from build123d import *

# Parameters (mm, degrees)
SKETCH_1_W      = 470
SKETCH_1_H      = 180
SKETCH_1_R      = 1.5
SKETCH_1_R_2    = 7
SKETCH_1_R_3    = 2
SKETCH_1_W_2    = 185
SKETCH_1_H_2    = 143
EXTRUDE_1_DEPTH = 5


with BuildPart() as part:
    # 草图1 → 凸台-拉伸1 (new body)
    with BuildSketch(Plane(origin=(0, 0, 0), x_dir=(1, 0, 0), z_dir=(0, 1, 0))):
        with Locations((0, 15)):
            Rectangle(SKETCH_1_W, SKETCH_1_H)
        with Locations((-96.5, 86)):
            Circle(SKETCH_1_R, mode=Mode.SUBTRACT)
        with Locations((96.5, 86)):
            Circle(SKETCH_1_R, mode=Mode.SUBTRACT)
        with Locations((96.5, -56)):
            Circle(SKETCH_1_R, mode=Mode.SUBTRACT)
        with Locations((-96.5, -56)):
            Circle(SKETCH_1_R, mode=Mode.SUBTRACT)
        with Locations((-125, 75)):
            Circle(SKETCH_1_R_2, mode=Mode.SUBTRACT)
        with Locations((-125, 45)):
            Circle(SKETCH_1_R_2, mode=Mode.SUBTRACT)
        with Locations((-125, 15)):
            Circle(SKETCH_1_R_2, mode=Mode.SUBTRACT)
        with Locations((-125, -15)):
            Circle(SKETCH_1_R_2, mode=Mode.SUBTRACT)
        with Locations((-125, -45)):
            Circle(SKETCH_1_R_2, mode=Mode.SUBTRACT)
        with Locations((-226, 35)):
            Circle(SKETCH_1_R, mode=Mode.SUBTRACT)
        with Locations((-186, 35)):
            Circle(SKETCH_1_R, mode=Mode.SUBTRACT)
        with Locations((-186, -5)):
            Circle(SKETCH_1_R, mode=Mode.SUBTRACT)
        with Locations((-226, -5)):
            Circle(SKETCH_1_R, mode=Mode.SUBTRACT)
        with Locations((-210, -50)):
            Circle(SKETCH_1_R_3, mode=Mode.SUBTRACT)
        with Locations((210, -50)):
            Circle(SKETCH_1_R_3, mode=Mode.SUBTRACT)
        with Locations((-210, 80)):
            Circle(SKETCH_1_R_3, mode=Mode.SUBTRACT)
        with Locations((210, 80)):
            Circle(SKETCH_1_R_3, mode=Mode.SUBTRACT)
        with Locations((0, 15)):
            Rectangle(SKETCH_1_W_2, SKETCH_1_H_2, mode=Mode.SUBTRACT)
    extrude(amount=EXTRUDE_1_DEPTH)


solid = part.part
Work out the finished part from the listing and answer in its coordinate system (mm). Round coordinates to 2 decimals unless told otherwise and drop trailing zeros. Order: outer loops, then holes, each group sorted by start corner. A loop starts at its lowest first (then second) coordinate and runs counter-clockwise, first axis right, second up. Notation, with made-up numbers: M -21,66 L -13,66 A10 ccw -13,82 Z; hole C -26.5,16 d7. An arc over 180 degrees is marked long. Put each result on its own line as item: value. Start each with the question number.
Q1. A flat-ended cylindrical pin translates along its axis: pin 1 (5 mm diameter, centred on x = 110.5, z = 35.5, fed in from -Y). Find the tip coordinate at first contact, or state that the pin passes through.
Q2. Section C-C, the plane y = 1.1 is taken. Give the number of separate pieces and of enclosed holes in the cut face, and give its area (3 significant figures).
Q3. Straight lines are drawn through the part: L1, parallel to X at y = 3.85, z = -86; L2, parallel to Z at x = 96.5, y = 1.25; L3, parallel to X at y = 2.65, z = 15. For each, find the intervals that lie inside material, in ascending order. Write a range as [from, to].
Q4. Section A-A, the plane z = 15 is taken. Write down the section's boundary in (x, y).
Q5. For a pull along Z with two mould halves and no side action, classify faces 1 (the flat face through (-3, 5, 64)), 2 (the cylindrical face through (-132, 2, 15)) as pulls with the +Z half, pulls with the -Z half, needs draft (parallel to the pull), parting line crosses it, or undercut.
Q6. Section B-B, the plane x = -22.5 is taken. Write down the section's boundary in (y, z), and give its area (3 significant figures).
Findings below:
1. pin 1: stops at y = 0
2. separate pieces: 1
2. enclosed holes: 18
2. area: 57,300 mm^2
3. L1: x = [-235, -98], [-95, -92.5], [92.5, 95], [98, 235]
3. L2: z = [-105, -87.5], [-84.5, 54.5], [57.5, 75]
3. L3: x = [-235, -132], [-118, -92.5], [92.5, 235]
4. outline: M -235,0 L -132,0 L -132,5 L -235,5 Z; M -118,0 L -92.5,0 L -92.5,5 L -118,5 Z; M 92.5,0 L 235,0 L 235,5 L 92.5,5 Z
5. face 1: needs draft
5. face 2: undercut
6. outline: M 0,-105 L 5,-105 L 5,-86.5 L 0,-86.5 Z; M 0,56.5 L 5,56.5 L 5,75 L 0,75 Z
6. area: 185 mm^2
